```python
from build123d import *

# Parameters (mm, degrees)
SKETCH1_W           = 200
SKETCH1_H           = 17.1
BOSS_EXTRUDE1_DEPTH = 4.7
CUT_EXTRUDE1_DEPTH  = 4.7
LPATTERN1_COUNT     = 6
LPATTERN1_PITCH     = 32
CUT_EXTRUDE2_DEPTH  = 4.7
LPATTERN2_COUNT     = 5
LPATTERN2_PITCH     = 32


with BuildPart() as part:
    # Sketch1 → Boss-Extrude1 (new body)
    with BuildSketch(Plane(origin=(0, 0, 0), x_dir=(1, 0, 0), z_dir=(0, 1, 0))):
        with Locations((100, 8.55)):
            Rectangle(SKETCH1_W, SKETCH1_H)
    extrude(amount=BOSS_EXTRUDE1_DEPTH)

    # Sketch2 → Cut-Extrude1 (cut)
    with BuildSketch(Plane(origin=(0, 4.7, 0), x_dir=(1, 0, 0), z_dir=(0, 1, 0))):
        with BuildLine():
            Line((26.789984467, 13.027698049), (14.324334337, 10.35))
            Line((14.324334337, 10.35), (19.388431138, 9.392177684))
            Line((19.388431138, 9.392177684), (27.210015533, 11.072301951))
            ThreePointArc((27.210015533, 11.072301951), (27.977698049, 12.260015533), (26.789984467, 13.027698049))
        make_face()
    cut_extrude1 = extrude(amount=-CUT_EXTRUDE1_DEPTH, mode=Mode.SUBTRACT)

    # LPattern1: Cut-Extrude1 ×6
    with Locations(*[(i * LPATTERN1_PITCH, 0, 0) for i in range(1, LPATTERN1_COUNT)]):
        add(cut_extrude1, mode=Mode.SUBTRACT)

    # Sketch3 → Cut-Extrude2 (cut)
    with BuildSketch(Plane(origin=(0, 4.7, 0), x_dir=(1, 0, 0), z_dir=(0, 1, 0))):
        with BuildLine():
            Line((42.817010597, 4.416885114), (30.282295805, 6.75))
            Line((30.282295805, 6.75), (35.318070317, 7.847030108))
            Line((35.318070317, 7.847030108), (43.182989403, 6.383114886))
            ThreePointArc((43.182989403, 6.383114886), (43.983114886, 5.217010597), (42.817010597, 4.416885114))
        make_face()
    cut_extrude2 = extrude(amount=-CUT_EXTRUDE2_DEPTH, mode=Mode.SUBTRACT)

    # LPattern2: Cut-Extrude2 ×5
    with Locations(*[(i * LPATTERN2_PITCH, 0, 0) for i in range(1, LPATTERN2_COUNT)]):
        add(cut_extrude2, mode=Mode.SUBTRACT)


solid = part.part
```
The listing builds one solid part. Answer for the finished solid, in the listing's coordinates (mm). A direction names the side the tool comes from. Give positions to 0.01 mm unless a question says otherwise; leave off trailing zeros. Loops run counter-clockwise (first coordinate to the right, second up) from the corner with the lowest first, then second, coordinate; pieces in that order, holes last. Notation, with made-up numbers: (14.25, 56.25) - (41.25, 56.25) arc R24 ccw to (41.25, 94.25) - close; hole circle Ø1 at (68.25, 39.25). An arc over 180 degrees is marked (long way). Answer as CSV lines item,"result". Start each with the question number.
Item 1: The mould has two halves that part along Z. Classify faces 1 (the face through (71.195, 2.383, -7.125)), 2 (the face through (99, 4.7, -9)): +Z half, -Z half, draft (parallel to the pull), parting line (faces both ways), or undercut.
Item 2: For faces 3 (the face through (200, 2, -8)), 4 (the face through (135.195, 2.383, -7.125)), determine the directions among +Z, -Z, +X, -X, +Y, -Y from which every point of the face is accessible in a straight line to the end or side of a thin tool.
Item 3: Find the intervals of material crossed by line 1 (Z direction, x = 50, y = 3.65); line 2 (Z direction, x = 54, y = 0.5), in increasing order. Write a range as from..to.
Item 4: A cutting plane is placed at A-A on y = 2.8. Count the separate pieces of the cut face and the enclosed holes in it, then the cut area to 3 significant figures.
Item 5: A cutting plane is placed at B-B on x = 54.5. Determine the outline of the cut face in (y, z), then the cut area to 3 significant figures.
Found:
1,face 1,"undercut"
1,face 2,"draft"
2,face 3,"+Z, -Z, +X, +Y, -Y"
2,face 4,"+Y, -Y"
3,line 1,"z = -17.1..-11.14, -9.65..0"
3,line 2,"z = -17.1..-12, -9.95..0"
4,separate pieces,"1"
4,enclosed holes,"11"
4,area,"3,170 mm^2"
5,outline,"(0, -17.1) - (4.7, -17.1) - (4.7, -12.11) - (0, -12.11) - close; (0, -10.06) - (4.7, -10.06) - (4.7, 0) - (0, 0) - close"
5,area,"70.8 mm^2"
